Build history of the part. All positions in model axes, mm. Give positions to 0.01 mm unless a question says otherwise; leave off trailing zeros. Loops run counter-clockwise (first coordinate to the right, second up) from the corner with the lowest first, then second, coordinate; pieces in that order, holes last. Notation, with made-up numbers: (29, -8) -> (56, -8) arc R27 ccw to (56, 10) -> close; hole circle Ø1 at (6.5, 69). An arc over 180 degrees is marked (long way). Answer as a JSON object with one key per item and string values. Group by question number.
Q1. Band-saw the part on B-B, the plane z = 131. Write the cut outline in (x, y).
Q2. Two-plate mould, pull along Y, no slides. Class faces 1 (the cylindrical face through (469.204, -5.749, 93.916)), 2 (the cylindrical face through (24.937, 393.712, 96.55)), 3 (the flat face through (292, -406.4, 94)), 4 (the flat face through (276, 6, 0)): pulls with the +Y half, pulls with the -Y half, needs draft (parallel to the pull), parting line crosses it, or undercut.
Q3. Wall check: probe 1 along Z at (x, y) = (48.5, -215); probe 2 along Z at (x, y) = (-19.5, 238.5); probe 3 along X at (y, z) = (-260, 146). Give the ranges that are in metal, low to high. Write a range as from..to.
Q4. Drop flat-ended pins along their axis: pin 1 (10 mm diameter, centred on y = -250, z = 49, fed in from +X); pin 2 (8 mm diameter, centred on y = 285, z = 64, fed in from -X); pin 3 (12 mm diameter, centred on y = -150, z = 167, fed in from +X). Give the stop position or say it passes through.
Q5. Band-saw the part on A-A, the plane z = 23. Write the cut outline in (x, y).
from build123d import *

# Parameters (mm, degrees)
F1_DEPTH = 190.5
F2_R     = 88.9


with BuildPart() as f1:
    # F0 (on Top) → F1 (new body)
    with BuildSketch(Plane.XY):
        with BuildLine():
            Line((0, -406.4), (0, 0))
            Line((0, 0), (0, 406.4))
            ThreePointArc((0, 406.4), (-50.8, 0), (0, -406.4))
        make_face()
        with BuildLine():
            Line((0, 406.4), (0, 0))
            Line((0, 0), (0, -406.4))
            Line((0, -406.4), (519.99896, -406.4))
            ThreePointArc((519.99896, -406.4), (469.19388, -0.000635), (519.9888, 406.4))
            Line((519.9888, 406.4), (0, 406.4))
        make_face()
    extrude(amount=F1_DEPTH)

    # F2
    f2_edges = [f1.edges().sort_by_distance(p)[0] for p in [
        (0, 406.4, 95.25),
        (0, -406.4, 95.25),
        (-50.8, 0, 0),
        (-50.8, 0, 190.5),
    ]]
    fillet(f2_edges, radius=F2_R)


solid = f1.part
Worked answers:
{
 "1": {"outline": "(-5.04, -364.04) arc R88.9 ccw to (70.71, -406.4) -> (520, -406.4) arc R1651 cw to (519.99, 406.4) -> (70.71, 406.4) arc R88.9 ccw to (-5.04, 364.04) arc R1646 ccw to start"},
 "2": {"face 1": "undercut", "face 2": "pulls with the +Y half", "face 3": "pulls with the -Y half", "face 4": "needs draft"},
 "3": {"probe 1": "0.11..190.39", "probe 2": "41.27..149.23", "probe 3": "-18.17..489.8"},
 "4": {"pin 1": "x = 489.01", "pin 2": "x = -23.71", "pin 3": "x = 476.58"},
 "5": {"outline": "(27.29, -395.08) arc R88.9 ccw to (70.71, -406.4) -> (520, -406.4) arc R1651 cw to (519.99, 406.4) -> (70.71, 406.4) arc R88.9 ccw to (27.29, 395.08) arc R1621.77 ccw to start"}
}
